The listing builds one solid part. Answer for the finished solid, in the listing's coordinates (mm). Face numbers are marked on the shaded views. A direction names the side the tool comes from. Round coordinates to 2 decimals unless told otherwise and drop trailing zeros. Order: outer loops, then holes, each group sorted by start corner. A loop starts at its lowest first (then second) coordinate and runs counter-clockwise, first axis right, second up. Notation, with made-up numbers: (63.5, -16.5) - (91.5, -16.5) arc R14 cw to (91.5, -7.5) - close; hole circle Ø5 at (89.5, -27.75). An arc over 180 degrees is marked (long way). Use CSV: the item, a comma, the result in double quotes. Start each with the question number.
Item 1: Find section C-C, the plane z = 50. Give the vertices of the cut face in (x, y), plus the area to 3 significant figures.
Item 2: Straight lines are drawn through the part: line 1 along Y through (x, z) = (44.75, 75); line 2 along Y through (x, z) = (-44, 25); line 3 along Y through (x, z) = (23, 94). For each, find the intervals that lie inside material, in ascending order. Write a range as [from, to].
Item 3: Determine the mould class of the marked faces 1, 2, 3 and 4 for opening direction X: +X half, -X half, draft (parallel to the pull), parting line (faces both ways), or undercut.
Item 4: Find section B-B, the plane y = 0. Give the vertices of the cut face in (x, z).
Item 5: Flat-ended cylindrical pins translate along their axes: P1, Ø18, axis at y = 25, z = 74.94, coming from the -X side; P2, Ø16, axis at y = -25, z = 25, coming from the +X side; P3, Ø16, axis at x = 25, y = -25, coming from the +Z side; P4, Ø16, axis at y = 20, z = 27, coming from the +X side. Find the tip coordinate at first contact, or state that the pin passes through.
Item 6: Find section A-A, the plane x = 43. Give the vertices of the cut face in (y, z), plus the area to 3 significant figures.
Item 7: Find section D-D, the plane x = 0. Give the vertices of the cut face in (y, z), plus the area to 3 significant figures.
Item 8: For the marked faces 5, 6 and 7, determine the directions among +Z, -Z, +X, -X, +Y, -Y from which every point of the face is accessible in a straight line to the end or side of a thin tool.
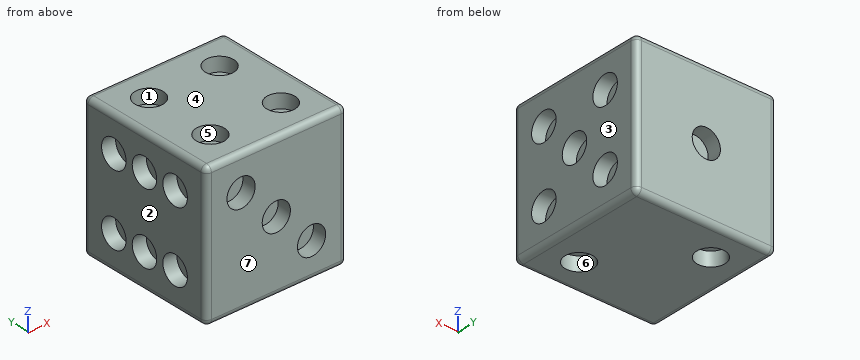
```python
from build123d import *

# Parameters (mm, degrees)
CROQUIS1_W              = 100
CROQUIS1_H              = 100
SALIENTE_EXTRUIR1_DEPTH = 100
CROQUIS8_R              = 10
CORTAR_EXTRUIR7_DEPTH   = 10
CORTAR_EXTRUIR9_START   = -10
CROQUIS10_R             = 10
CORTAR_EXTRUIR9_DEPTH   = 10
CROQUIS11_R             = 10
CORTAR_EXTRUIR11_DEPTH  = 10
CORTAR_EXTRUIR12_START  = -10
CROQUIS9_R              = 10
CORTAR_EXTRUIR12_DEPTH  = 10
CROQUIS12_R             = 10
CORTAR_EXTRUIR13_DEPTH  = 10
CORTAR_EXTRUIR14_START  = -10
CROQUIS13_R             = 10
CORTAR_EXTRUIR14_DEPTH  = 10
REDONDEO2_R             = 4
REDONDEO3_R             = 4


with BuildPart() as part:
    # Croquis1 → Saliente-Extruir1 (new body)
    with BuildSketch(Plane.XY):
        Rectangle(CROQUIS1_W, CROQUIS1_H)
    extrude(amount=SALIENTE_EXTRUIR1_DEPTH)

    # Croquis8 → Cortar-Extruir7 (cut)
    with BuildSketch(Plane(origin=(0, 50, 0), x_dir=(1, 0, 0), z_dir=(0, 1, 0))):
        with Locations(Location((0, -50, 0), (0, 0, 270))):
            Circle(CROQUIS8_R)
    extrude(amount=-CORTAR_EXTRUIR7_DEPTH, mode=Mode.SUBTRACT)

    # Croquis10 → Cortar-Extruir9 (cut)
    with BuildSketch(Plane.XZ.offset(50).offset(CORTAR_EXTRUIR9_START)):
        with Locations(Location((-25, 75, 0), (0, 0, 270))):
            Circle(CROQUIS10_R)
        with Locations(Location((0, 50, 0), (0, 0, 90))):
            Circle(CROQUIS10_R)
        with Locations(Location((25, 25, 0), (0, 0, 270))):
            Circle(CROQUIS10_R)
    extrude(amount=CORTAR_EXTRUIR9_DEPTH, mode=Mode.SUBTRACT)

    # Croquis11 → Cortar-Extruir11 (cut)
    with BuildSketch(Plane(origin=(0, 0, 0), x_dir=(-1, 0, 0), z_dir=(0, 0, -1))):
        with Locations((-25, -25)):
            Circle(CROQUIS11_R)
        with Locations((25, 25)):
            Circle(CROQUIS11_R)
    extrude(amount=-CORTAR_EXTRUIR11_DEPTH, mode=Mode.SUBTRACT)

    # Croquis9 → Cortar-Extruir12 (cut)
    with BuildSketch(Plane.XY.offset(100).offset(CORTAR_EXTRUIR12_START)):
        with Locations(Location((-25, 25, 0), (0, 0, 180))):
            Circle(CROQUIS9_R)
        with Locations(Location((25, -25, 0), (0, 0, 180))):
            Circle(CROQUIS9_R)
        with Locations((25, 25)):
            Circle(CROQUIS9_R)
        with Locations((-25, -25)):
            Circle(CROQUIS9_R)
    extrude(amount=CORTAR_EXTRUIR12_DEPTH, mode=Mode.SUBTRACT)

    # Croquis12 → Cortar-Extruir13 (cut)
    with BuildSketch(Plane(origin=(50, 0, 0), x_dir=(0, 0, -1), z_dir=(1, 0, 0))):
        with Locations((-25, -25)):
            Circle(CROQUIS12_R)
        with Locations((-50, 0)):
            Circle(CROQUIS12_R)
        with Locations((-75, -25)):
            Circle(CROQUIS12_R)
        with Locations((-75, 25)):
            Circle(CROQUIS12_R)
        with Locations((-25, 25)):
            Circle(CROQUIS12_R)
    extrude(amount=-CORTAR_EXTRUIR13_DEPTH, mode=Mode.SUBTRACT)

    # Croquis13 → Cortar-Extruir14 (cut)
    with BuildSketch(Plane.ZY.offset(50).offset(CORTAR_EXTRUIR14_START)):
        with Locations(Location((25, 25, 0), (0, 0, 180))):
            Circle(CROQUIS13_R)
        with Locations((25, 0)):
            Circle(CROQUIS13_R)
        with Locations(Location((25, -25, 0), (0, 0, 180))):
            Circle(CROQUIS13_R)
        with Locations((74.939373622, 25)):
            Circle(CROQUIS13_R)
        with Locations((74.939373622, 0)):
            Circle(CROQUIS13_R)
        with Locations((74.939373622, -25)):
            Circle(CROQUIS13_R)
    extrude(amount=CORTAR_EXTRUIR14_DEPTH, mode=Mode.SUBTRACT)

    # Redondeo2
    redondeo2_edges = [part.edges().sort_by_distance(p)[0] for p in [
        (0, -50, 100),
        (50, 0, 100),
        (50, -50, 50),
    ]]
    fillet(redondeo2_edges, radius=REDONDEO2_R)

    # Redondeo3
    redondeo3_edges = [part.edges().sort_by_distance(p)[0] for p in [
        (-50, -48.828427125, 98.828427125),
        (48.828427125, 50, 98.828427125),
        (-50, 2, 100),
        (-2, -50, 0),
        (-50, 0, 0),
        (0, 50, 0),
        (-50, 50, 50),
        (50, 2, 0),
        (50, 50, 48),
        (48.828427125, -48.828427125, 0),
        (-50, -50, 48),
        (-2, 50, 100),
    ]]
    fillet(redondeo3_edges, radius=REDONDEO3_R)


solid = part.part
```
Worked out:
1,outline,"(-50, -46) arc R4 ccw to (-46, -50) - (-10, -50) - (-10, -40) - (10, -40) - (10, -50) - (46, -50) arc R4 ccw to (50, -46) - (50, -10) - (40, -10) - (40, 10) - (50, 10) - (50, 46) arc R4 ccw to (46, 50) - (10, 50) - (10, 40) - (-10, 40) - (-10, 50) - (-46, 50) arc R4 ccw to (-50, 46) - close"
1,area,"9,390 mm²"
2,line 1,"y = [-50, -35], [-15, 15], [35, 50]"
2,line 2,"y = [-50, -35], [-15, -10], [10, 15], [35, 50]"
2,line 3,"y = [-50, -34.8], [-15.2, 15.2], [34.8, 50]"
3,face 1,"undercut"
3,face 2,"-X half"
3,face 3,"+X half"
3,face 4,"draft"
4,outline,"(-50, 4) arc R4 ccw to (-46, 0) - (46, 0) arc R4 ccw to (50, 4) - (50, 40) - (40, 40) - (40, 60) - (50, 60) - (50, 96) arc R4 ccw to (46, 100) - (-46, 100) arc R4 ccw to (-50, 96) - (-50, 84.94) - (-40, 84.94) - (-40, 64.94) - (-50, 64.94) - (-50, 35) - (-40, 35) - (-40, 15) - (-50, 15) - close"
5,P1,"stops at x = -40"
5,P2,"stops at x = 40"
5,P3,"stops at z = 90"
5,P4,"stops at x = 50"
6,outline,"(-50, 4) arc R4 ccw to (-46, 0) - (46, 0) arc R4 ccw to (50, 4) - (50, 96) arc R4 ccw to (46, 100) - (-46, 100) arc R4 ccw to (-50, 96) - close; hole circle Ø20 at (-25, 25); hole circle Ø20 at (-25, 75); hole circle Ø20 at (0, 50); hole circle Ø20 at (25, 25); hole circle Ø20 at (25, 75)"
6,area,"8,420 mm²"
7,outline,"(-50, 4) arc R4 ccw to (-46, 0) - (46, 0) arc R4 ccw to (50, 4) - (50, 40) - (40, 40) - (40, 60) - (50, 60) - (50, 96) arc R4 ccw to (46, 100) - (-46, 100) arc R4 ccw to (-50, 96) - (-50, 60) - (-40, 60) - (-40, 40) - (-50, 40) - close"
7,area,"9,590 mm²"
8,face 5,"+Z"
8,face 6,"-Z"
8,face 7,"+Z, -Z, +X, -X, -Y"
